Source: CAD feature listing. Evaluate the final solid. Frame: model axes, mm. A direction names the side the tool comes from. Give positions to 0.01 mm unless a question says otherwise; leave off trailing zeros. Order: outer loops, then holes, each group sorted by start corner. A loop starts at its lowest first (then second) coordinate and runs counter-clockwise, first axis right, second up. Notation, with made-up numbers: M 13,69.5 L 49,69.5 A15 ccw 49,76.5 Z; hole C 29.5,83.25 d8. An arc over 180 degrees is marked long. Return JSON: item names as keys, results as strings.
from build123d import *

# Parameters (mm, degrees)
SKETCH1_R           = 15
BOSS_EXTRUDE1_DEPTH = 3
SKETCH2_R           = 15
SKETCH2_R_2         = 12.5
BOSS_EXTRUDE2_DEPTH = 17
SKETCH3_R           = 3
SKETCH3_R_2         = 1.5
CUT_EXTRUDE1_DEPTH  = 3
BOSS_EXTRUDE3_DEPTH = 20
SKETCH6_W           = 13
SKETCH6_H           = 13
CUT_EXTRUDE3_DEPTH  = 26
SKETCH7_R           = 2
CUT_EXTRUDE4_DEPTH  = 58.905178378


with BuildPart() as part:
    # Sketch1 → Boss-Extrude1 (new body)
    with BuildSketch(Plane.XY):
        Circle(SKETCH1_R)
    extrude(amount=BOSS_EXTRUDE1_DEPTH)

    # Sketch2 → Boss-Extrude2 (add)
    with BuildSketch(Plane.XY.offset(3)):
        Circle(SKETCH2_R)
        Circle(SKETCH2_R_2, mode=Mode.SUBTRACT)
    extrude(amount=BOSS_EXTRUDE2_DEPTH)

    # Sketch3 → Cut-Extrude1 (cut)
    with BuildSketch(Plane.XY.offset(3)):
        Circle(SKETCH3_R)
        with Locations((-6.960222154, -4.87906831)):
            Circle(SKETCH3_R_2)
        with Locations((6.960222154, 4.87906831)):
            Circle(SKETCH3_R_2)
    extrude(amount=-CUT_EXTRUDE1_DEPTH, mode=Mode.SUBTRACT)

    # Sketch4 → Boss-Extrude3 (add)
    with BuildSketch(Plane(origin=(0, 0, 0), x_dir=(-1, 0, 0), z_dir=(0, 0, -1))):
        with BuildLine():
            Line((14.487171628, 3.888683351), (41.81162802, -15.265574417))
            Line((41.81162802, -15.265574417), (28.609443183, -34.099116715))
            Line((28.609443183, -34.099116715), (1.284986791, -14.944858947))
            ThreePointArc((1.284986791, -14.944858947), (12.282744977, -8.610120546), (14.487171628, 3.888683351))
        make_face()
    extrude(amount=-BOSS_EXTRUDE3_DEPTH)

    # Sketch6 → Cut-Extrude3 (cut)
    with BuildSketch(Plane(origin=(-35.210535602, -24.682345566, 0), x_dir=(-0.5740080364217665, 0.8188496651542504, 0), z_dir=(-0.8188496651542504, -0.5740080364217665, 0))):
        with Locations((0, -10)):
            Rectangle(SKETCH6_W, SKETCH6_H)
    extrude(amount=-CUT_EXTRUDE3_DEPTH, mode=Mode.SUBTRACT)

    # Sketch7 → Cut-Extrude4 (cut, through all)
    with BuildSketch(Plane(origin=(6.601092419, -9.416771149, 0), x_dir=(0, 0, 1), z_dir=(0.5740080364217666, -0.8188496651542504, 0))):
        with Locations(Location((10, 37.7, 0), (0, 0, 270))):
            Circle(SKETCH7_R)
        with Locations(Location((10, 22.2, 0), (0, 0, 270))):
            Circle(SKETCH7_R)
    extrude(amount=-CUT_EXTRUDE4_DEPTH, mode=Mode.SUBTRACT)


solid = part.part
1. Section query C-C (y = -1.5). Return loops of the section in (x, z), then the cut area to 3 significant figures.
Evaluation:
{"outline": "M -22.17,0 L -2.6,0 L -2.6,3 L -12.41,3 L -12.41,20 L -22.17,20 Z; M 2.6,0 L 14.92,0 L 14.92,20 L 12.41,20 L 12.41,3 L 2.6,3 Z", "area": "304 mm^2"}
2. Section query D-D (y = 11.5). Return loops of the section in (x, z).
Evaluation:
{"outline": "M -9.63,0 L 9.63,0 L 9.63,20 L 4.9,20 L 4.9,3 L -4.9,3 L -4.9,20 L -9.63,20 Z"}
3. Section query B-B (z = 6). Return loops of the section in (x, y).
Evaluation:
{"outline": "M -41.81,-15.27 L -38.94,-19.36 L -17.65,-4.44 L -10.19,-15.08 L -31.48,-30 L -28.61,-34.1 L -1.28,-14.94 A15 ccw long -14.49,3.89 Z; hole C 0,0 d25"}
4. First-contact query: pin 1 (7.5 mm diameter, centred on x = -26, y = -13.5, fed in from -Z); pin 2 (10 mm diameter, centred on x = -31.5, z = 14, fed in from +Y); pin 3 (12.5 mm diameter, centred on x = 5, y = -2, fed in from +Z); pin 4 (8 mm diameter, centred on y = -9.5, z = 2.5, fed in from -X). Flat tips, straight axial feed; report the tip coordinate or a pass-through.
Evaluation:
{"pin 1": "stops at z = 0", "pin 2": "stops at y = -4.53", "pin 3": "stops at z = 3", "pin 4": "stops at x = -39.29"}
5. Ray query, probe 1 along Y at (x, z) = (0, 8.5); probe 2 along Z at (x, y) = (-32.5, -26); probe 3 along Y at (x, z) = (0, 1.9). Return the intervals inside material, ascending.
Evaluation:
{"probe 1": "y = -15 to -12.5, 12.5 to 15", "probe 2": "z = 0 to 3.5, 16.5 to 20", "probe 3": "y = -15 to -3, 3 to 15"}
6. Draft query along Y for faces 1 (the face through (-8.15, -5.79, 1.52)), 2 (the face through (-15.138, -24.656, 9.86)), 3 (the face through (-27.958, -5.554, 9.86)). Return one class per face: pulls with the +Y half, pulls with the -Y half, needs draft (parallel to the pull), parting line crosses it, or undercut.
Evaluation:
{"face 1": "undercut", "face 2": "pulls with the -Y half", "face 3": "pulls with the +Y half"}
7. Set-up query: faces 4 (the face through (3, -3, 3)), 5 (the face through (12.55, 8.216, 9.86)), 6 (the face through (-25, -17, 3.5)). Return all of +Z, -Z, +X, -X, +Y, -Y with unobstructed straight access to the full face (end or side cutting, diameter ignored); none if empty.
Evaluation:
{"face 4": "+Z", "face 5": "+Z, -Z", "face 6": "none"}
8. Section query A-A (x = 0). Return loops of the section in (y, z).
Evaluation:
{"outline": "M -15,0 L -3,0 L -3,3 L -12.5,3 L -12.5,20 L -15,20 Z; M 3,0 L 15,0 L 15,20 L 12.5,20 L 12.5,3 L 3,3 Z"}
